Source: three-view drawing plus pictorial views. Frame: mm from the lowest corner of the part. A direction names the side the tool comes from. Give positions to 0.01 mm unless a question says otherwise; leave off trailing zeros. Loops run counter-clockwise (first coordinate to the right, second up) from the corner with the lowest first, then second, coordinate; pieces in that order, holes last. Notation, with made-up numbers: M -33.5,80 L 15.5,80 A17 cw 15.5,92 Z; hole C 56.5,-36.75 d3. An arc over 180 degrees is marked long. Answer as a JSON object with one key per item and string values. Group by question number.
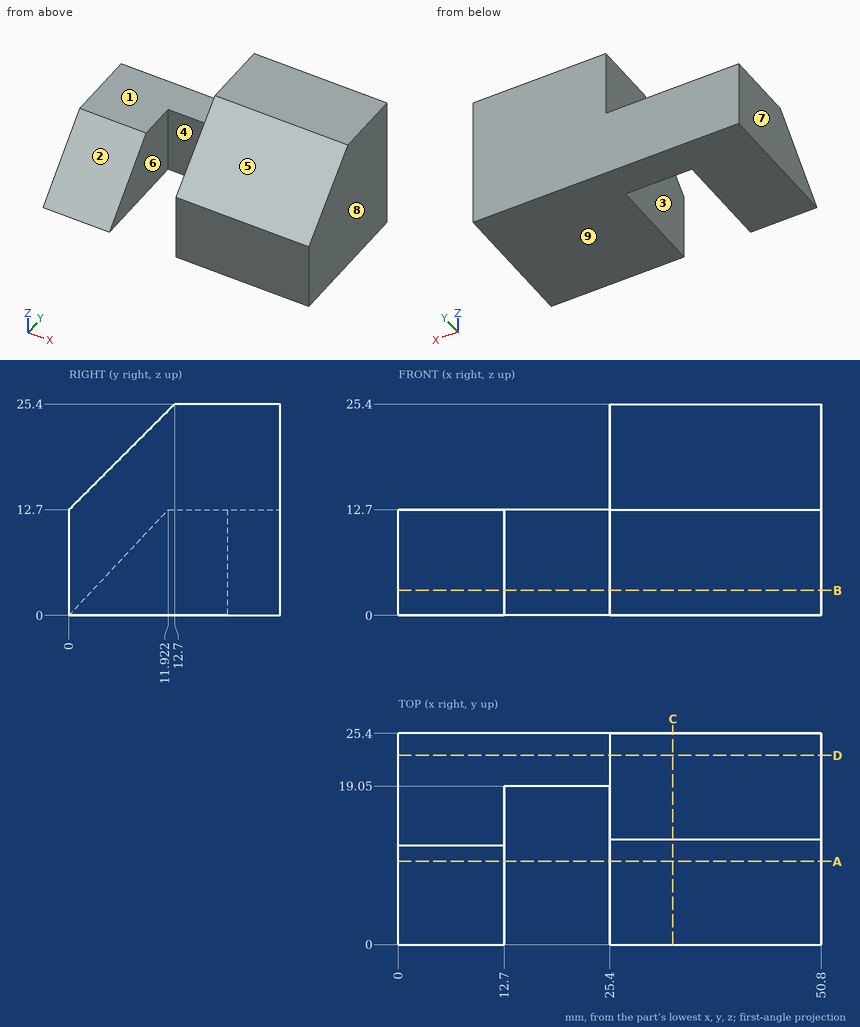
1. Material intervals for L1, parallel to X at y = 18.25, z = 8.5; L2, parallel to X at y = 10.75, z = 16; L3, parallel to Y at x = 21.5, z = 1.5, sorted ascending.
2. Section B-B (z = 3). Output: boundary loops of the cut face in (x, y), then the cut area to 3 significant figures.
3. Section A-A (y = 10). Output: boundary loops of the cut face in (x, z).
4. Section D-D (y = 22.75). Output: boundary loops of the cut face in (x, z), then the cut area to 3 significant figures.
5. Mould query, pull axis X, two halves, no side actions, for the marked faces 6, 7, 8 and 9. Classes: pulls with the +X half, pulls with the -X half, needs draft (parallel to the pull), parting line crosses it, or undercut.
6. Section C-C (x = 33). Output: boundary loops of the cut face in (y, z).
7. First-contact query: P1, Ø1, axis at x = 24.5, y = 17, coming from the -Z side; P2, Ø12, axis at y = 6, z = 21, coming from the +X side; P3, Ø4, axis at x = 18, z = 5, coming from the -Y side; P4, Ø4, axis at x = 17, y = 20, coming from the +Z side. Flat tips, straight axial feed; report the tip coordinate or a pass-through.
8. Reachability of the marked faces 1, 2, 3, 4 and 5 from +Z, -Z, +X, -X, +Y, -Y: full face, straight path, thin tool, end or side. Return the list, or none.
Geometry results:
{
 "1": {"L1": "0 to 12.7, 25.4 to 50.8", "L2": "25.4 to 50.8", "L3": "19.05 to 25.4"},
 "2": {"outline": "M 0,2.82 L 12.7,2.82 L 12.7,19.05 L 25.4,19.05 L 25.4,0 L 50.8,0 L 50.8,25.4 L 0,25.4 Z", "area": "1,010 mm2"},
 "3": {"outline": "M 0,0 L 12.7,0 L 12.7,10.65 L 0,10.65 Z; M 25.4,0 L 50.8,0 L 50.8,22.7 L 25.4,22.7 Z"},
 "4": {"outline": "M 0,0 L 50.8,0 L 50.8,25.4 L 25.4,25.4 L 25.4,12.7 L 0,12.7 Z", "area": "968 mm2"},
 "5": {"face 6": "undercut", "face 7": "pulls with the -X half", "face 8": "pulls with the +X half", "face 9": "needs draft"},
 "6": {"outline": "M 0,0 L 25.4,0 L 25.4,25.4 L 12.7,25.4 L 0,12.7 Z"},
 "7": {"P1": "through", "P2": "x = 50.8", "P3": "y = 19.05", "P4": "z = 12.7"},
 "8": {"face 1": "+Z, -X, +Y, -Y", "face 2": "+Z, -X, -Y", "face 3": "+Z, -Y", "face 4": "+Z, -Z, -Y", "face 5": "+Z, +X, -X, -Y"}
}
